Model file for the job. Use its own axes, mm. Give positions to 0.01 mm unless a question says otherwise; leave off trailing zeros. Loops run counter-clockwise (first coordinate to the right, second up) from the corner with the lowest first, then second, coordinate; pieces in that order, holes last. Notation, with made-up numbers: M -33.75,-22 L 0.25,-22 A27 ccw 0.25,9 Z; hole C 38.25,29.25 d5. An arc over 180 degrees is marked long. Answer in a Markdown table with one row per item.
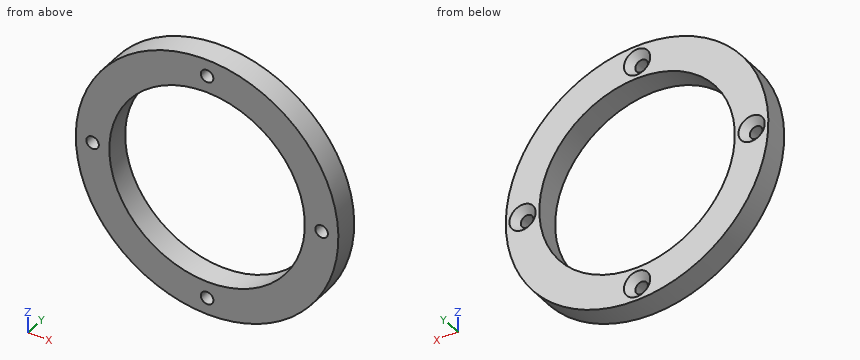
```python
from build123d import *

# Parameters (mm, degrees)
SKETCH1_R                                       = 47
SKETCH1_R_2                                     = 35
BOSS_EXTRUDE1_DEPTH                             = 8.6
CSK_FOR_M4_FLAT_HEAD_MACHINE_SCREW1_D           = 4.5
CSK_FOR_M4_FLAT_HEAD_MACHINE_SCREW1_CSINK_D     = 9.4
CSK_FOR_M4_FLAT_HEAD_MACHINE_SCREW1_CSINK_ANGLE = 90


with BuildPart() as part:
    # Sketch1 → Boss-Extrude1 (new body)
    with BuildSketch(Plane(origin=(0, 0, 0), x_dir=(1, 0, 0), z_dir=(0, 1, 0))):
        with Locations(Location((0, 0, 0), (0, 0, 90))):
            Circle(SKETCH1_R)
        with Locations(Location((0, 0, 0), (0, 0, 90))):
            Circle(SKETCH1_R_2, mode=Mode.SUBTRACT)
    extrude(amount=BOSS_EXTRUDE1_DEPTH)

    # CSK for M4 Flat Head Machine Screw1 (through all)
    with Locations(Plane(origin=(0, 8.6, 0), x_dir=(1, 0, 0), z_dir=(0, 1, 0))):
        with Locations((0, 41), (0, -41), (-41, 0), (41, 0)):
            CounterSinkHole(CSK_FOR_M4_FLAT_HEAD_MACHINE_SCREW1_D / 2, CSK_FOR_M4_FLAT_HEAD_MACHINE_SCREW1_CSINK_D / 2, counter_sink_angle=CSK_FOR_M4_FLAT_HEAD_MACHINE_SCREW1_CSINK_ANGLE)


solid = part.part
```
(1) Wall check: L1, parallel to Z at x = 32.5, y = 2.5; L2, parallel to X at y = 8, z = 27; L3, parallel to X at y = 1, z = -29. Give the ranges that are in metal, low to high.
Established:
| item | result |
|---|---|
| L1 | z = -33.95 to -12.99, 12.99 to 33.95 |
| L2 | x = -38.47 to -22.27, 22.27 to 38.47 |
| L3 | x = -36.99 to -19.6, 19.6 to 36.99 |
(2) Saw through at A-A, the plane x = 0. Give the cut face in (y, z).
Established:
| item | result |
|---|---|
| outline | M 0,-47 L 8.6,-47 L 8.6,-45.7 L 6.15,-43.25 L 0,-43.25 Z; M 0,-38.75 L 6.15,-38.75 L 8.6,-36.3 L 8.6,-35 L 0,-35 Z; M 0,35 L 8.6,35 L 8.6,36.3 L 6.15,38.75 L 0,38.75 Z; M 0,43.25 L 6.15,43.25 L 8.6,45.7 L 8.6,47 L 0,47 Z |
(3) Saw through at C-C, the plane z = -30. Give the cut face in (x, y).
Established:
| item | result |
|---|---|
| outline | M -36.18,0 L -18.03,0 L -18.03,8.6 L -36.18,8.6 Z; M 18.03,0 L 36.18,0 L 36.18,8.6 L 18.03,8.6 Z |
(4) Saw through at D-D, the plane x = -41. Give the cut face in (y, z).
Established:
| item | result |
|---|---|
| outline | M 0,-22.98 L 8.6,-22.98 L 8.6,-4.7 L 6.15,-2.25 L 0,-2.25 Z; M 0,2.25 L 6.15,2.25 L 8.6,4.7 L 8.6,22.98 L 0,22.98 Z |
(5) Saw through at B-B, the plane z = 0. Give the cut face in (x, y).
Established:
| item | result |
|---|---|
| outline | M -47,0 L -43.25,0 L -43.25,6.15 L -45.7,8.6 L -47,8.6 Z; M -38.75,0 L -35,0 L -35,8.6 L -36.3,8.6 L -38.75,6.15 Z; M 35,0 L 38.75,0 L 38.75,6.15 L 36.3,8.6 L 35,8.6 Z; M 43.25,0 L 47,0 L 47,8.6 L 45.7,8.6 L 43.25,6.15 Z |
(6) Flat gauge pins, fed straight in: P1, Ø2, axis at y = 7, z = 7, coming from the +X side; P2, Ø7, axis at x = -41, z = 0, coming from the -Y side; P3, Ø5, axis at x = 10.5, y = 4, coming from the +Z side. Where does each tip first touch, or does it go through?
Established:
| item | result |
|---|---|
| P1 | stops at x = 46.62 |
| P2 | stops at y = 0 |
| P3 | stops at z = 46.31 |
